Geometry check sheet. Reference: the model listing, model coordinates, mm. A direction names the side the tool comes from. Give positions to 0.01 mm unless a question says otherwise; leave off trailing zeros. Loops run counter-clockwise (first coordinate to the right, second up) from the corner with the lowest first, then second, coordinate; pieces in that order, holes last.
1. Cross-section at C-C, the plane z = 10.5. Record the cut outline in (x, y).
2. Tool access check on faces 1 (the cylindrical face through (61.99, 2.85, 6.08)), 2 (the flat face through (44, 42, 12)), 3 (the flat face through (-22.5, 42, 14)). Record the directions out of +Z, -Z, +X, -X, +Y, -Y that give a thin tool (end or side, any length) a straight path to the whole face; none if there is none.
3. Go/stop test with flat-tipped pins: pin 1 Ø16 at (x, y) = (-52.5, 72.5) entering from +Z; pin 2 Ø1.2 at (y, z) = (30, 13) entering from +X. Record where each tip stops, or that it passes through.
4. Release check for a two-part mould opening along X. For faces 4 (the flat face through (-65, 42, 6)), 5 (the flat face through (1, 42, 0)), 6 (the flat face through (65, 42, 6)), 7 (the cylindrical face through (-57.495, 12.72, 5.916)) record: +X half, -X half, draft (parallel to the pull), parting line (faces both ways), or undercut.
5. Material ranges on L1, parallel to Y at x = 52.5, z = 6.5; L2, parallel to Y at x = 48.5, z = 9.25; L3, parallel to Z at x = -33, y = 32.5, recorded low to high.
6. Cross-section at B-B, the plane x = 52.5. Record the cut outline in (y, z).
7. Cross-section at A-A, the plane y = 72.5. Record the cut outline in (x, z), plus the area to 3 significant figures.
8. Cross-section at D-D, the plane y = 19.5. Record the cut outline in (x, z).
from build123d import *

# Parameters (mm, degrees)
EXTRUDE1_DEPTH          = 85
M10X1_25_TAPPED_HOLE1_D = 10
FILLET1_R               = 10
FILLET1_OF_MIRROR1_R    = 10


with BuildPart() as part:
    # Sketch1 → Extrude1 (new body)
    with BuildSketch(Plane(origin=(0, 0, 0), x_dir=(1, 0, 0), z_dir=(0, 1, 0))):
        Polygon((0, 0), (65, 0), (65, -12), (22.5, -12), (22.5, -16), (0, -16), align=None)
    extrude1 = extrude(amount=EXTRUDE1_DEPTH)

    # M10x1.25 Tapped Hole1 (through all)
    with Locations(Plane.XY.offset(12)):
        with Locations((52.5, 12.5), (52.5, 72.5)):
            m10x1_25_tapped_hole1 = Hole(M10X1_25_TAPPED_HOLE1_D / 2)

    # Fillet1
    fillet1_edges = [part.edges().sort_by_distance(p)[0] for p in [
        (65, 85, 6),
        (65, 0, 6),
    ]]
    fillet(fillet1_edges, radius=FILLET1_R)

    # Mirror1: Extrude1, M10x1.25 Tapped Hole1 across plane
    add(extrude1.mirror(Plane(origin=(0, 0, 0), x_dir=(0, 0, 1), z_dir=(1, 0, 0))))
    add(m10x1_25_tapped_hole1.mirror(Plane(origin=(0, 0, 0), x_dir=(0, 0, 1), z_dir=(1, 0, 0))), mode=Mode.SUBTRACT)

    # Fillet1 of Mirror1
    fillet1_of_mirror1_edges = [part.edges().sort_by_distance(p)[0] for p in [
        (-65, 85, 6),
        (-65, 0, 6),
    ]]
    fillet(fillet1_of_mirror1_edges, radius=FILLET1_OF_MIRROR1_R)


solid = part.part
Result:
1. outline: (-65, 10) arc R10 ccw to (-55, 0) - (55, 0) arc R10 ccw to (65, 10) - (65, 75) arc R10 ccw to (55, 85) - (-55, 85) arc R10 ccw to (-65, 75) - close; hole circle Ø10 at (-52.5, 12.5); hole circle Ø10 at (-52.5, 72.5); hole circle Ø10 at (52.5, 12.5); hole circle Ø10 at (52.5, 72.5)
2. face 1: +Z, -Z, +X, -Y
2. face 2: +Z, +X, +Y, -Y
2. face 3: +Z, -X, +Y, -Y
3. pin 1: stops at z = 12
3. pin 2: stops at x = 22.5
4. face 4: -X half
4. face 5: draft
4. face 6: +X half
4. face 7: undercut
5. L1: y = 0 to 7.5, 17.5 to 67.5, 77.5 to 85
5. L2: y = 0 to 9.5, 15.5 to 69.5, 75.5 to 85
5. L3: z = 0 to 12
6. outline: (0, 0) - (7.5, 0) - (7.5, 12) - (0, 12) - close; (17.5, 0) - (67.5, 0) - (67.5, 12) - (17.5, 12) - close; (77.5, 0) - (85, 0) - (85, 12) - (77.5, 12) - close
7. outline: (-65, 0) - (-57.5, 0) - (-57.5, 12) - (-65, 12) - close; (-47.5, 0) - (47.5, 0) - (47.5, 12) - (22.5, 12) - (22.5, 16) - (-22.5, 16) - (-22.5, 12) - (-47.5, 12) - close; (57.5, 0) - (65, 0) - (65, 12) - (57.5, 12) - close
7. area: 1,500 mm2
8. outline: (-65, 0) - (65, 0) - (65, 12) - (22.5, 12) - (22.5, 16) - (-22.5, 16) - (-22.5, 12) - (-65, 12) - close
